Could you check a few things on this model? Use its own coordinates, in mm. A direction names the side the tool comes from. Give positions to 0.01 mm unless a question says otherwise; leave off trailing zeros. Order: outer loops, then holes, each group sorted by start corner. A loop starts at its lowest first (then second) coordinate and runs counter-clockwise, first axis right, second up. Notation, with made-up numbers: M 37,-36.75 L 93,-36.75 A16 cw 93,-12.75 Z; hole C -37,-33.5 d2. An arc over 180 degrees is marked long. Answer in a Markdown table with one row per item. Add a question column.
```python
from build123d import *

# Parameters (mm, degrees)
BOSS_EXTRUDE1_DEPTH                               = 5
CSK_FOR_M3_FLAT_HEAD_MACHINE_SCREW1_D             = 3.6
CSK_FOR_M3_FLAT_HEAD_MACHINE_SCREW1_CSINK_D       = 6.3
CSK_FOR_M3_FLAT_HEAD_MACHINE_SCREW1_CSINK_ANGLE   = 90
SKETCH16_R                                        = 1.8
CUT_EXTRUDE7_DEPTH                                = 2.1
MIRROR6_COPY_1_DEPTH                              = 5
MIRROR6_COPY_2_D                                  = 3.6
MIRROR6_COPY_2_CSINK_D                            = 6.3
MIRROR6_COPY_2_CSINK_ANGLE                        = 90
MIRROR6_COPY_3_SKETCH_R                           = 1.8
MIRROR6_COPY_3_DEPTH                              = 2.1
SKETCH6_R                                         = 12.5
CUT_EXTRUDE2_DEPTH                                = 0.75
SKETCH6_4_R                                       = 12.5
SKETCH6_4_W                                       = 5
SKETCH6_4_H                                       = 3.5
CUT_EXTRUDE5_DEPTH                                = 0.75
CSK_FOR_M2_5_FLAT_HEAD_MACHINE_SCREW3_D           = 3.1
CSK_FOR_M2_5_FLAT_HEAD_MACHINE_SCREW3_CSINK_D     = 5.5
CSK_FOR_M2_5_FLAT_HEAD_MACHINE_SCREW3_CSINK_ANGLE = 90
CIRPATTERN1_COUNT                                 = 3


with BuildPart() as part:
    # Sketch1 → Boss-Extrude1 (new body)
    with BuildSketch(Plane(origin=(0, 0, 0), x_dir=(1, 0, 0), z_dir=(0, 1, 0))):
        with BuildLine():
            Line((-16.25, 26.25), (-16.25, 16.25))
            Line((-16.25, 16.25), (-2.25, 16.25))
            Line((-2.25, 16.25), (-2.25, 26.25))
            ThreePointArc((-2.25, 26.25), (-9.25, 33.25), (-16.25, 26.25))
        make_face()
        Polygon((-2.25, 16.25), (-16.25, 16.25), (-16.25, -16.25), (16.25, -16.25), (16.25, 16.25), align=None)
    boss_extrude1 = extrude(amount=BOSS_EXTRUDE1_DEPTH)

    # CSK for M3 Flat Head Machine Screw1 (through all)
    with Locations(Plane.XZ):
        with Locations((-9.25, -24.75)):
            csk_for_m3_flat_head_machine_screw1 = CounterSinkHole(CSK_FOR_M3_FLAT_HEAD_MACHINE_SCREW1_D / 2, CSK_FOR_M3_FLAT_HEAD_MACHINE_SCREW1_CSINK_D / 2, counter_sink_angle=CSK_FOR_M3_FLAT_HEAD_MACHINE_SCREW1_CSINK_ANGLE)

    # Sketch16 → Cut-Extrude7 (cut)
    with BuildSketch(Plane(origin=(0, 5, 0), x_dir=(1, 0, 0), z_dir=(0, 1, 0))):
        with BuildLine():
            Line((-5.829108303, 27.75), (-12.670891697, 27.75))
            ThreePointArc((-12.670891697, 27.75), (-13.8, 24.75), (-12.670891697, 21.75))
            Line((-12.670891697, 21.75), (-5.829108303, 21.75))
            ThreePointArc((-5.829108303, 21.75), (-4.991622538, 23.147276883), (-4.7, 24.75))
            ThreePointArc((-4.7, 24.75), (-4.991622538, 26.352723117), (-5.829108303, 27.75))
        make_face()
        with Locations(Location((-9.25, 24.75, 0), (0, 0, 90))):
            Circle(SKETCH16_R, mode=Mode.SUBTRACT)
    cut_extrude7 = extrude(amount=-CUT_EXTRUDE7_DEPTH, mode=Mode.SUBTRACT)

    # Mirror2: Boss-Extrude1, CSK for M3 Flat Head Machine Screw1, Cut-Extrude7 across plane
    add(boss_extrude1.mirror(Plane(origin=(0, 0, 0), x_dir=(0, 0, 1), z_dir=(1, 0, 0))))
    add(csk_for_m3_flat_head_machine_screw1.mirror(Plane(origin=(0, 0, 0), x_dir=(0, 0, 1), z_dir=(1, 0, 0))), mode=Mode.SUBTRACT)
    add(cut_extrude7.mirror(Plane(origin=(0, 0, 0), x_dir=(0, 0, 1), z_dir=(1, 0, 0))), mode=Mode.SUBTRACT)

    # Mirror6: Boss-Extrude1, CSK for M3 Flat Head Machine Screw1, Cut-Extrude7 across plane
    add(boss_extrude1.mirror(Plane.XY))
    add(csk_for_m3_flat_head_machine_screw1.mirror(Plane.XY), mode=Mode.SUBTRACT)
    add(cut_extrude7.mirror(Plane.XY), mode=Mode.SUBTRACT)

    # Mirror6 copy 1 sketch → Mirror6 copy 1 (add)
    with BuildSketch(Plane(origin=(0, 0, 0), x_dir=(-1, 0, 0), z_dir=(0, 1, 0))):
        with BuildLine():
            Line((-16.25, 26.25), (-16.25, 16.25))
            Line((-16.25, 16.25), (-2.25, 16.25))
            Line((-2.25, 16.25), (-2.25, 26.25))
            ThreePointArc((-2.25, 26.25), (-9.25, 33.25), (-16.25, 26.25))
        make_face()
        Polygon((-2.25, 16.25), (-16.25, 16.25), (-16.25, -16.25), (16.25, -16.25), (16.25, 16.25), align=None)
    extrude(amount=MIRROR6_COPY_1_DEPTH)

    # Mirror6 copy 2 (through all)
    with Locations(Plane(origin=(0, 0, 0), x_dir=(-1, 0, 0), z_dir=(0, -1, 0))):
        with Locations((-9.25, -24.75)):
            CounterSinkHole(MIRROR6_COPY_2_D / 2, MIRROR6_COPY_2_CSINK_D / 2, counter_sink_angle=MIRROR6_COPY_2_CSINK_ANGLE)

    # Mirror6 copy 3 sketch → Mirror6 copy 3 (cut)
    with BuildSketch(Plane(origin=(0, 5, 0), x_dir=(-1, 0, 0), z_dir=(0, 1, 0))):
        with BuildLine():
            Line((-5.829108303, 27.75), (-12.670891697, 27.75))
            ThreePointArc((-12.670891697, 27.75), (-13.8, 24.75), (-12.670891697, 21.75))
            Line((-12.670891697, 21.75), (-5.829108303, 21.75))
            ThreePointArc((-5.829108303, 21.75), (-4.991622538, 23.147276883), (-4.7, 24.75))
            ThreePointArc((-4.7, 24.75), (-4.991622538, 26.352723117), (-5.829108303, 27.75))
        make_face()
        with Locations(Location((-9.25, 24.75, 0), (0, 0, 90))):
            Circle(MIRROR6_COPY_3_SKETCH_R, mode=Mode.SUBTRACT)
    extrude(amount=-MIRROR6_COPY_3_DEPTH, mode=Mode.SUBTRACT)

    # Sketch6 → Cut-Extrude2 (cut)
    with BuildSketch(Plane(origin=(0, 5, 0), x_dir=(1, 0, 0), z_dir=(0, 1, 0))):
        with Locations(Location((0, 0, 0), (0, 0, 270))):
            Circle(SKETCH6_R)
    extrude(amount=-CUT_EXTRUDE2_DEPTH, mode=Mode.SUBTRACT)

    # Sketch6<4> → Cut-Extrude5 (cut)
    with BuildSketch(Plane(origin=(0, 5, 0), x_dir=(1, 0, 0), z_dir=(0, 1, 0))):
        Circle(SKETCH6_4_R)
        with Locations((0, 12.5)):
            Rectangle(SKETCH6_4_W, SKETCH6_4_H)
    cut_extrude5 = extrude(amount=-CUT_EXTRUDE5_DEPTH, mode=Mode.SUBTRACT)

    # CSK for M2.5 Flat Head Machine Screw3 (through all)
    with Locations(Plane.XZ):
        with Locations((0, -10.25)):
            csk_for_m2_5_flat_head_machine_screw3 = CounterSinkHole(CSK_FOR_M2_5_FLAT_HEAD_MACHINE_SCREW3_D / 2, CSK_FOR_M2_5_FLAT_HEAD_MACHINE_SCREW3_CSINK_D / 2, counter_sink_angle=CSK_FOR_M2_5_FLAT_HEAD_MACHINE_SCREW3_CSINK_ANGLE)

    # CirPattern1: Cut-Extrude5, CSK for M2.5 Flat Head Machine Screw3 ×3 about axis
    cirpattern1_axis = Axis((0, 0, 0), (0, 1, 0))
    add([cut_extrude5.rotate(cirpattern1_axis, i * 360 / CIRPATTERN1_COUNT) for i in range(1, CIRPATTERN1_COUNT)], mode=Mode.SUBTRACT)
    add([csk_for_m2_5_flat_head_machine_screw3.rotate(cirpattern1_axis, i * 360 / CIRPATTERN1_COUNT) for i in range(1, CIRPATTERN1_COUNT)], mode=Mode.SUBTRACT)


solid = part.part
```
1. Will these pins go through, and if not, where does the flat tip stop? P1, Ø4, axis at x = 9.25, z = -24.75, coming from the +Y side; P2, Ø6.5, axis at x = -7, z = -23.5, coming from the +Y side; P3, Ø4.5, axis at x = 9.25, z = 24.75, coming from the -Y side; P4, Ø1.5, axis at x = -3.5, y = 2, coming from the +Z side.
2. Suppose I cut it at A-A on z = 17. List the corners of the cut face in (x, y) for me, plus the area to 3 significant figures.
3. For faces 1 (the flat face through (-9, 4, 21.75)), 2 (the flat face through (2.25, 2, 21)), 3 (the cylindrical face through (-9.1, 2.46, -33.25)), which set-ups out of +Z, -Z, +X, -X, +Y, -Y let a thin tool reach every point of the face, with its end or its side?
4. If I drill on line 1 along X through (y, z) = (1.7, -24.75); line 2 along X through (y, z) = (2.3, 21); line 3 along Z through (x, y) = (11, 0.35), over which ranges is the centre line in solid material (lowest first)? Write a range as [from, to].
5. Suppose I cut it at C-C on z = -10.25. List the corners of the cut face in (x, y) for me.
6. Thinking about a two-plate mould opening in X: for faces 4 (the cylindrical face through (13.8, 4, -24.8)), 5 (the flat face through (16.25, 2, 0)), which applies, pulls with the +X half, pulls with the -X half, needs draft (parallel to the pull), parting line crosses it, or undercut?
7. Suppose I cut it at B-B on x = 0. List the corners of the cut face in (y, z) for me, plus the area to 3 significant figures.
8. Suppose I cut it at D-D on x = 14.5. List the corners of the cut face in (y, z) for me.
Findings below:
| question | item | result |
|---|---|---|
| 1 | P1 | y = 2.9 |
| 1 | P2 | y = 5 |
| 1 | P3 | y = 0.9 |
| 1 | P4 | z = 31.15 |
| 2 | outline | M -16.25,0 L -2.25,0 L -2.25,5 L -16.25,5 Z; M 2.25,0 L 16.25,0 L 16.25,5 L 2.25,5 Z |
| 2 | area | 140 mm2 |
| 3 | face 1 | +Y |
| 3 | face 2 | +Z, +Y, -Y |
| 3 | face 3 | -Z, +Y, -Y |
| 4 | line 1 | [-16.25, -11.05], [-7.45, -2.25], [2.25, 7.45], [11.05, 16.25] |
| 4 | line 2 | [-16.25, -2.25], [2.25, 16.25] |
| 4 | line 3 | [-33.03, -26.94], [-22.56, 4.01], [6.24, 22.56], [26.94, 33.03] |
| 5 | outline | M -16.25,0 L -2.75,0 L -1.55,1.2 L -1.55,4.25 L -7.15,4.25 L -7.15,5 L -16.25,5 Z; M 1.55,1.2 L 2.75,0 L 16.25,0 L 16.25,5 L 7.15,5 L 7.15,4.25 L 1.55,4.25 Z |
| 6 | face 4 | undercut |
| 6 | face 5 | pulls with the +X half |
| 7 | outline | M 0,-16.25 L 5,-16.25 L 5,-14.25 L 4.25,-14.25 L 4.25,-11.8 L 1.2,-11.8 L 0,-13 Z; M 0,-7.5 L 1.2,-8.7 L 4.25,-8.7 L 4.25,12.5 L 5,12.5 L 5,16.25 L 0,16.25 Z |
| 7 | area | 128 mm2 |
| 8 | outline | M 0,-30.88 L 5,-30.88 L 5,30.88 L 0,30.88 Z |
